Can you work these out from the drawing? Everything is in mm from the part's minimum corner. Round coordinates to 2 decimals unless told otherwise and drop trailing zeros. Loops run counter-clockwise (first coordinate to the right, second up) from the corner with the lowest first, then second, coordinate; pieces in that order, holes last. Notation, with made-up numbers: (36, 38) -> (62, 38) arc R26 cw to (62, 69) -> close; hole circle Ø1 at (64.25, -14). An arc over 180 degrees is marked (long way). Use CSV: the item, a comma, the result in double quotes. Start each with the question number.
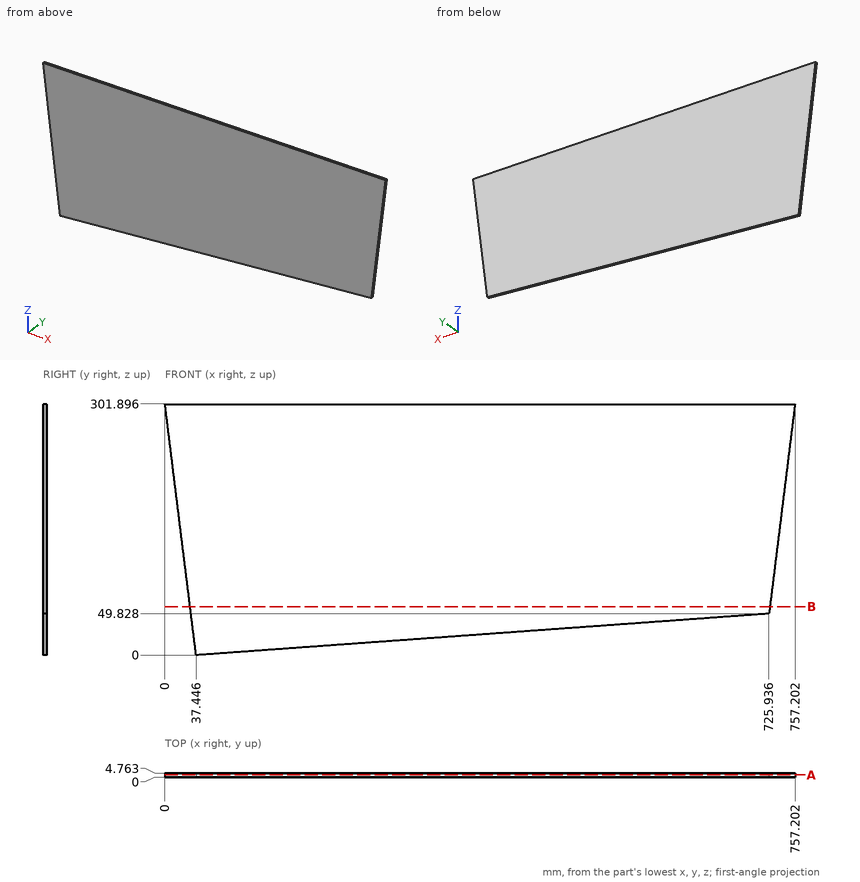
1. Suppose I cut it at A-A (y = 2.75). List the corners of the cut face in (x, z) for me (1 decimal).
2. Will this pin go through, and if not, where does the flat tip stop? pin 1 (1.5 mm diameter, centred on x = 173, y = 1.5, fed in from -Z).
3. Suppose I cut it at B-B (z = 58.5). List the corners of the cut face in (x, y) for me, then the cut area to 3 significant figures.
4. If I drill on L1, parallel to X at y = 3.4, z = 261; L2, parallel to Z at x = 723, y = 4.5 (1 decimal); L3, parallel to X at y = 1.9, z = 276, over which ranges is the centre line in solid material (lowest first)?
Geometry check:
1,outline,"(0, 301.9) -> (37.4, 0) -> (725.9, 49.8) -> (757.2, 301.9) -> close"
2,pin 1,"stops at z = 9.76"
3,outline,"(30.19, 0) -> (727.01, 0) -> (727.01, 4.76) -> (30.19, 4.76) -> close"
3,area,"3,320 mm²"
4,L1,"x = 5.07 to 752.13"
4,L2,"z = 49.6 to 301.9"
4,L3,"x = 3.21 to 753.99"
